Design review of the part shown in the three views and the two pictorial views. Dimensions are in mm from the part's minimum x, y and z. Round coordinates to 2 decimals unless told otherwise and drop trailing zeros. Loops run counter-clockwise (first coordinate to the right, second up) from the corner with the lowest first, then second, coordinate; pieces in that order, holes last. Notation, with made-up numbers: M 45,55 L 57,55 A14 cw 57,66 Z; hole C -32,86.25 d5. An arc over 180 degrees is marked long. Return JSON: item names as keys, results as strings. Group by question number.
Q1. Consider section C-C (z = 686). State the section outline as (x, y) points, and give its area (3 significant figures).
Q2. Clearance check with flat-ended pins moving along their axes: pin 1 Ø6 at (x, y) = (463.5, 15) entering from -Z; pin 2 Ø12 at (x, y) = (375.5, 63) entering from -Z; pin 3 Ø3 at (y, z) = (48, 194) entering from -X (1 decimal). State where each tip first meets the part, or that it passes through.
Q3. Consider section D-D (x = 423). State the section outline as (y, z) points.
Q4. Draft analysis for pull direction Z (two halves, no side actions). For the marked faces 1 and 2, state which applies: pulls with the +Z half, pulls with the -Z half, needs draft (parallel to the pull), parting line crosses it, or undercut.
Q5. To check wall thickness, follow line 1 along X through (y, z) = (45, 599); line 2 along X through (y, z) = (39, 634.5) (1 decimal); line 3 along Z through (x, y) = (422.5, 16) (1 decimal). State the ranges of each line that lie inside material, in increasing order.
Q6. Consider section A-A (x = 71). State the section outline as (y, z) points (1 decimal), and give its area (3 significant figures).
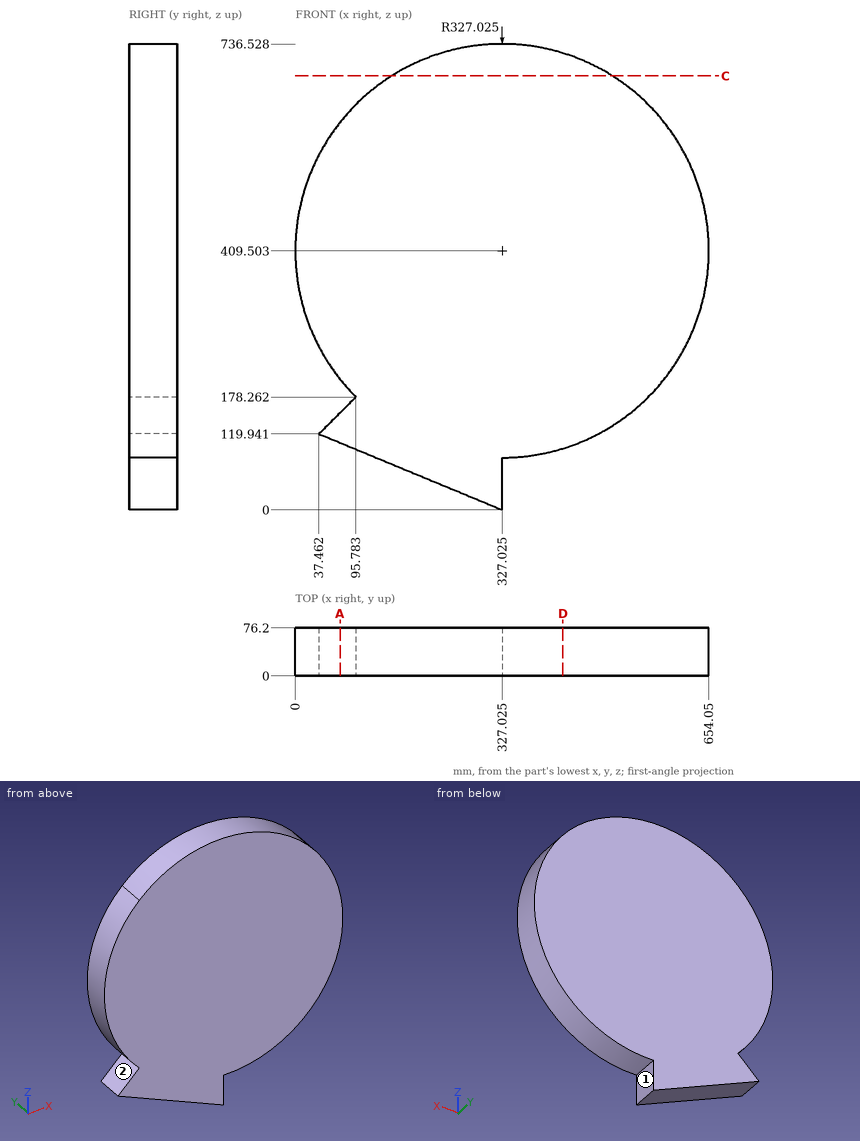
Values:
{
 "1": {"outline": "M 152.4,0 L 501.65,0 L 501.65,76.2 L 152.4,76.2 Z", "area": "26,600 mm2"},
 "2": {"pin 1": "stops at z = 110.96", "pin 2": "stops at z = 85.25", "pin 3": "stops at x = 79.7"},
 "3": {"outline": "M 0,96.88 L 76.2,96.88 L 76.2,722.13 L 0,722.13 Z"},
 "4": {"face 1": "needs draft", "face 2": "undercut"},
 "5": {"line 1": "x = 60.5 to 593.55", "line 2": "x = 89.7 to 564.3", "line 3": "z = 96.7 to 722.3"},
 "6": {"outline": "M 0,106 L 76.2,106 L 76.2,153.5 L 0,153.5 Z; M 0,206 L 76.2,206 L 76.2,613 L 0,613 Z", "area": "34,600 mm2"}
}
